from build123d import *

# Parameters (mm, degrees)
SKETCH1_R                                    = 41
SKETCH1_R_2                                  = 21.05
BOSS_EXTRUDE1_DEPTH                          = 3.175
SKETCH2_R                                    = 23
CUT_EXTRUDE1_DEPTH                           = 1.5
CSK_FOR_M4_COUNTERSUNK_FLAT_HEAD_SCR_2_COUNT = 2
CSK_FOR_M4_COUNTERSUNK_FLAT_HEAD_SCR_2_PITCH = 38
CSK_FOR_M4_COUNTERSUNK_FLAT_HEAD_SCR_3_COUNT = 2
CSK_FOR_M4_COUNTERSUNK_FLAT_HEAD_SCR_3_PITCH = 65.817930688
CSK_FOR_M4_COUNTERSUNK_FLAT_HEAD_SCR_4_COUNT = 2
CSK_FOR_M4_COUNTERSUNK_FLAT_HEAD_SCR_4_PITCH = 76
CSK_FOR_M4_COUNTERSUNK_FLAT_HEAD_SCR_5_COUNT = 2
CSK_FOR_M4_COUNTERSUNK_FLAT_HEAD_SCR_5_PITCH = 65.817930688
CSK_FOR_M4_COUNTERSUNK_FLAT_HEAD_SCR_6_COUNT = 2
CSK_FOR_M4_COUNTERSUNK_FLAT_HEAD_SCR_6_PITCH = 38
CSK_FOR_M4_COUNTERSUNK_FLAT_HEAD_SCR_7_COUNT = 2
CSK_FOR_M4_COUNTERSUNK_FLAT_HEAD_SCR_7_PITCH = 38
SKETCH5_R                                    = 3.1
CUT_EXTRUDE2_DEPTH                           = 59.069618924


with BuildPart() as part:
    # Sketch1 → Boss-Extrude1 (new body)
    with BuildSketch(Plane(origin=(0, 0, 0), x_dir=(0, 1, 0), z_dir=(0, 0, 1))):
        with Locations(Location((0, 0, 0), (0, 0, 270))):
            Circle(SKETCH1_R)
        with Locations(Location((0, 0, 0), (0, 0, 270))):
            Circle(SKETCH1_R_2, mode=Mode.SUBTRACT)
    extrude(amount=BOSS_EXTRUDE1_DEPTH)

    # Sketch2 → Cut-Extrude1 (cut)
    with BuildSketch(Plane(origin=(0, 0, 0), x_dir=(1, 0, 0), z_dir=(0, 0, -1))):
        with Locations(Location((0, 0, 0), (0, 0, 180))):
            Circle(SKETCH2_R)
    extrude(amount=-CUT_EXTRUDE1_DEPTH, mode=Mode.SUBTRACT)

    # Sketch4 → CSK for M4 Countersunk Flat Head Screw1 (revolve, cut)
    with BuildSketch(Plane(origin=(0, 38, 3.175), x_dir=(0, -1, 0), z_dir=(1, 0, 0))):
        Polygon((0, 0), (0, 3.175), (2.25, 3.175), (2.25, 2.45), (4.7, 0), align=None)
    csk_for_m4_countersunk_flat_head_screw1 = revolve(axis=Axis((0, 38, 9.525), (0, 0, -1)), mode=Mode.SUBTRACT)

    # CSK for M4 Countersunk Flat Head Scr 2: CSK for M4 Countersunk Flat Head Screw1 ×2
    with Locations(*[Vector(0.8660254037844387, -0.49999999999999994, 0) * (i * CSK_FOR_M4_COUNTERSUNK_FLAT_HEAD_SCR_2_PITCH) for i in range(1, CSK_FOR_M4_COUNTERSUNK_FLAT_HEAD_SCR_2_COUNT)]):
        add(csk_for_m4_countersunk_flat_head_screw1, mode=Mode.SUBTRACT)

    # CSK for M4 Countersunk Flat Head Scr 3: CSK for M4 Countersunk Flat Head Screw1 ×2
    with Locations(*[Vector(0.5000000000000001, -0.8660254037844386, 0) * (i * CSK_FOR_M4_COUNTERSUNK_FLAT_HEAD_SCR_3_PITCH) for i in range(1, CSK_FOR_M4_COUNTERSUNK_FLAT_HEAD_SCR_3_COUNT)]):
        add(csk_for_m4_countersunk_flat_head_screw1, mode=Mode.SUBTRACT)

    # CSK for M4 Countersunk Flat Head Scr 4: CSK for M4 Countersunk Flat Head Screw1 ×2
    with Locations(*[(0, -i * CSK_FOR_M4_COUNTERSUNK_FLAT_HEAD_SCR_4_PITCH, 0) for i in range(1, CSK_FOR_M4_COUNTERSUNK_FLAT_HEAD_SCR_4_COUNT)]):
        add(csk_for_m4_countersunk_flat_head_screw1, mode=Mode.SUBTRACT)

    # CSK for M4 Countersunk Flat Head Scr 5: CSK for M4 Countersunk Flat Head Screw1 ×2
    with Locations(*[Vector(-0.49999999999999983, -0.8660254037844388, 0) * (i * CSK_FOR_M4_COUNTERSUNK_FLAT_HEAD_SCR_5_PITCH) for i in range(1, CSK_FOR_M4_COUNTERSUNK_FLAT_HEAD_SCR_5_COUNT)]):
        add(csk_for_m4_countersunk_flat_head_screw1, mode=Mode.SUBTRACT)

    # CSK for M4 Countersunk Flat Head Scr 6: CSK for M4 Countersunk Flat Head Screw1 ×2
    with Locations(*[Vector(-0.8660254037844387, -0.4999999999999999, 0) * (i * CSK_FOR_M4_COUNTERSUNK_FLAT_HEAD_SCR_6_PITCH) for i in range(1, CSK_FOR_M4_COUNTERSUNK_FLAT_HEAD_SCR_6_COUNT)]):
        add(csk_for_m4_countersunk_flat_head_screw1, mode=Mode.SUBTRACT)

    # CSK for M4 Countersunk Flat Head Scr 7: CSK for M4 Countersunk Flat Head Screw1 ×2
    with Locations(*[(0, -i * CSK_FOR_M4_COUNTERSUNK_FLAT_HEAD_SCR_7_PITCH, 0) for i in range(1, CSK_FOR_M4_COUNTERSUNK_FLAT_HEAD_SCR_7_COUNT)]):
        add(csk_for_m4_countersunk_flat_head_screw1, mode=Mode.SUBTRACT)

    # Sketch5 → Cut-Extrude2 (cut, through all)
    with BuildSketch(Plane.XY.offset(3.175)):
        with Locations((-27.715000373, -3.984815472)):
            Circle(SKETCH5_R)
        with Locations((-21.160988082, -18.33610055)):
            Circle(SKETCH5_R)
        with Locations((-7.888511592, -26.865803261)):
            Circle(SKETCH5_R)
        with Locations((7.888511592, -26.865803261)):
            Circle(SKETCH5_R)
        with Locations((21.160988082, -18.33610055)):
            Circle(SKETCH5_R)
        with Locations((27.715000373, -3.984815472)):
            Circle(SKETCH5_R)
        with Locations((25.46969587, 11.631620364)):
            Circle(SKETCH5_R)
        with Locations((15.137942889, 23.555098919)):
            Circle(SKETCH5_R)
        with Locations((0, 28)):
            Circle(SKETCH5_R)
        with Locations((-15.137942889, 23.555098919)):
            Circle(SKETCH5_R)
        with Locations((-25.46969587, 11.631620364)):
            Circle(SKETCH5_R)
    extrude(amount=-CUT_EXTRUDE2_DEPTH, mode=Mode.SUBTRACT)


solid = part.part
Design review of the part built by this model. Coordinates are the model's own, in mm. A direction names the side the tool comes from. Round coordinates to 2 decimals unless told otherwise and drop trailing zeros. Order: outer loops, then holes, each group sorted by start corner. A loop starts at its lowest first (then second) coordinate and runs counter-clockwise, first axis right, second up. Notation, with made-up numbers: M 80,-40 L 126,-40 A23 ccw 126,-4 Z; hole C 28.25,83 d11. An arc over 180 degrees is marked long. Answer as CSV lines item,"result". Start each with the question number.
1) The part is to be moulded in two halves that separate along X. For faces 3 (the face through (-18.204, -17.405, 1.61)), 4 (the face through (-10, 19, 3.175)), say which applies: +X half, -X half, draft (parallel to the pull), parting line (faces both ways), or undercut.
2) Add section A-A (x = -8.5). Give the boundary of the cut face in (y, z) (3 decimals).
3) Add section C-C (x = 0). Give the boundary of the cut face in (y, z) (3 decimals).
4) Tool access review of faces 1 (the face through (-0.404, 31.074, 1.61)), 2 (the face through (2.994, 22.804, 0.74)): name each direction out of +Z, -Z, +X, -X, +Y, -Y from which nothing blocks a thin tool from reaching the whole face with its end or side.
5) For pin 1 Ø5 at (x, y) = (-7.89, -26.87) entering from -Z; pin 2 Ø1 at (y, z) = (-16, 0.5) entering from -X, all flat-tipped, find the tip position at first contact; note any pin that passes through.
6) Add section D-D (z = 2.3). Give the number of separate pieces and of enclosed holes in the cut face, then the cut area to 3 significant figures.
7) Wall thickness on line 1 along Y through (x, z) = (0, 0.2); line 2 along X through (y, z) = (-19, 0.45); line 3 along Y through (x, z) = (12.5, 1.15): over which ranges is each line inside the solid? List them lowest first. Write a range as [from, to].
8) Add section B-B (y = 6). Give the boundary of the cut face in (x, z) (3 decimals), then the cut area to 3 significant figures.
Resolved:
1,face 3,"undercut"
1,face 4,"draft"
2,outline,"M -40.109,0 L -29.905,0 L -29.905,3.175 L -40.109,3.175 Z; M -23.827,0 L -21.372,0 L -21.372,1.5 L -19.258,1.5 L -19.258,3.175 L -23.827,3.175 Z; M 19.258,1.5 L 21.372,1.5 L 21.372,0 L 40.109,0 L 40.109,3.175 L 19.258,3.175 Z"
3,outline,"M -41,0 L -40.25,0 L -40.25,0.725 L -41,1.475 Z; M -35.75,0 L -23,0 L -23,1.5 L -21.05,1.5 L -21.05,3.175 L -33.3,3.175 L -35.75,0.725 Z; M 21.05,1.5 L 23,1.5 L 23,0 L 24.9,0 L 24.9,3.175 L 21.05,3.175 Z; M 31.1,0 L 35.75,0 L 35.75,0.725 L 33.3,3.175 L 31.1,3.175 Z; M 40.25,0 L 41,0 L 41,1.475 L 40.25,0.725 Z"
4,face 1,"+Z, -Z"
4,face 2,"-Z"
5,pin 1,"through"
5,pin 2,"x = -37.96"
6,separate pieces,"1"
6,enclosed holes,"12"
6,area,"3,300 mm^2"
7,line 1,"[-41, -40.25], [-35.75, -23], [23, 24.9], [31.1, 35.75], [40.25, 41]"
7,line 2,"[-36.33, -35.16], [-30.66, -24.19], [-18.13, -12.96], [12.96, 18.13], [24.19, 30.66], [35.16, 36.33]"
7,line 3,"[-39.05, -19.31], [19.31, 21.93], [25.18, 39.05]"
8,outline,"M -40.559,0 L -22.204,0 L -22.204,1.5 L -20.177,1.5 L -20.177,3.175 L -40.559,3.175 Z; M 20.177,1.5 L 22.204,1.5 L 22.204,0 L 40.559,0 L 40.559,3.175 L 20.177,3.175 Z"
8,area,"123 mm^2"
